Autodesk Fusion 360 part; units mm, degrees
sketch "Esboço1" plane through (0, 0, 0) normal (0, 0, 1) x (1, 0, 0)
  line L0 (16.7794, 7) -> (68.3114, 7)
  line L1 (68.3114, 7) -> (68.3114, 13)
  line L2 (68.3114, 13) -> (16.7794, 13)
  line L3 (16.7794, 13) -> (16.7794, 7)
  circle A0 centre (20.7794, 10) radius 1.6
  circle A1 centre (64.3114, 10) radius 1.6
  dimension "d1" = 3.2
  dimension "d2" = 3.2
  dimension "d3" = 43.532
  dimension "d4" = 4
  dimension "d6" = 6
  dimension "d7" = 3
  dimension "d14" = 4
extrude "Extrusão1" add sketch "Esboço1" along normal blind 4 makes body 1
fillet "Arredondamento1" radius 3 2 edges at (16.7794, 13, 2) (16.7794, 7, 2) on bodies 1
fillet "Arredondamento2" radius 3 2 edges at (68.3114, 13, 2) (68.3114, 7, 2) on bodies 1
copy_body "Corpo -> Componente1" bodies 1 removing the originals makes body 2 in component "Component"
scale "Escala1" factor 0.7 about (65.3114, 13, 4) bodies 2 in component "Component"
scale "Escala2" factor 1.14 about (33.439, 8.8, 1.2) bodies 2 in component "Component"
component "Component" placed x (1, 0, 0) y (0, 1, 0) z (0, 0, 1) at (0, 0, 0)
For this review, take the finished solid that the model builds, in its own axes (mm). Give positions to 0.01 mm unless a question says otherwise; leave off trailing zeros. Order: outer loops, then holes, each group sorted by start corner. A loop starts at its lowest first (then second) coordinate and runs counter-clockwise, first axis right, second up. Notation, with made-up numbers: M 62,-13 L 109,-13 A28 ccw 109,15 Z; hole C 61,-26 d11. An arc over 180 degrees is marked long. Answer in a Markdown table with one row per item. Add a question column.
(1) Consider section D-D on y = 11.85. State the section outline as (x, z) points, and give its area (3 significant figures).
(2) Wall thickness on probe 1 along X at (y, z) = (11.05, 2.15); probe 2 along X at (y, z) = (10.8, 3.1); probe 3 along Y at (x, z) = (35, 1.4): over which ranges is each line inside the solid? List them lowest first. Write a range as [from, to].
(3) Mouldability with a two-part tool opening along Y and no side actions: class faces 1 (the face through (35.455, 10.81, 2.774)), 2 (the face through (71.485, 12.868, 2.818)), 3 (the face through (51, 11, 4.392)), 4 (the face through (71.448, 9.483, 2.818)) as +Y half, -Y half, draft (parallel to the pull), parting line (faces both ways), or undercut.
(4) Consider section C-C on z = 1.9. Give the number of separate pieces and of enclosed holes in the cut face, and give its area (3 significant figures).
(5) Consider section B-B on x = 34. State the section outline as (y, z) points.
(6) Consider section A-A on y = 10.35. State the section outline as (x, z) points.
Evaluation:
| question | item | result |
|---|---|---|
| 1 | outline | M 31.14,1.2 L 33.14,1.2 L 33.14,4.39 L 31.14,4.39 Z; M 35.33,1.2 L 67.88,1.2 L 67.88,4.39 L 35.33,4.39 Z; M 70.07,1.2 L 72.08,1.2 L 72.08,4.39 L 70.07,4.39 Z |
| 1 | area | 117 mm^2 |
| 2 | probe 1 | x = [31.05, 32.97], [35.51, 67.71], [70.24, 72.16] |
| 2 | probe 2 | x = [31.08, 33.02], [35.45, 67.76], [70.19, 72.13] |
| 2 | probe 3 | y = [8.8, 10.17], [12.22, 13.59] |
| 3 | face 1 | undercut |
| 3 | face 2 | +Y half |
| 3 | face 3 | draft |
| 3 | face 4 | -Y half |
| 4 | separate pieces | 1 |
| 4 | enclosed holes | 2 |
| 4 | area | 182 mm^2 |
| 5 | outline | M 8.8,1.2 L 9.94,1.2 L 9.94,4.39 L 8.8,4.39 Z; M 12.45,1.2 L 13.59,1.2 L 13.59,4.39 L 12.45,4.39 Z |
| 6 | outline | M 31.2,1.2 L 33.28,1.2 L 33.28,4.39 L 31.2,4.39 Z; M 35.2,1.2 L 68.02,1.2 L 68.02,4.39 L 35.2,4.39 Z; M 69.93,1.2 L 72.01,1.2 L 72.01,4.39 L 69.93,4.39 Z |
